Autodesk Inventor part; units mm, degrees
ref_plane "Płaszczyzna konstrukcyjna1" through (-3.5034, 3, 0) normal (0, 0, 1) x (1, 0, 0)
ref_plane "YZ Plane" through (0, 0, 0) normal (1, 0, 0) x (0, 1, 0)
ref_plane "XZ Plane" through (0, 0, 0) normal (0, 1, 0) x (-1, 0, 0)
sketch "Szkic1" plane through (0, 0, 0) normal (0, 1, 0) x (-1, 0, 0)
  line L0 (42.918, 0) -> (-17.7038, -35)
  line L1 (-17.7038, -35) -> (-17.7038, 35)
  line L2 (-17.7038, 35) -> (42.918, 0)
  point P0 (0, 0)
  dimension "d0" = 70
  dimension "d1" = 35
  dimension "d2" = 60
  dimension "d3" = 60
extrude "Wyciągnięcie proste1" add sketch "Szkic1" along normal blind 3
fillet "Zaokrąglenie1" radius 7 3 edges at (17.7038, 1.5, 35) (17.7038, 1.5, -35) (-42.918, 1.5, 0)
sketch "Szkic2" plane through (0, 3, 0) normal (0, 1, 0) x (1, 0, 0)
  circle A0 centre (10.92, -22.8756) radius 2.5
  arc A1 (7.2038, -28.9378) -> (17.7038, -22.8756) centre (10.7038, -22.8756) ccw
  circle A2 centre (-28.918, 0) radius 2.5
  circle A3 centre (10.7038, 23.0617) radius 2.5
  arc A4 (-32.418, 6.0622) -> (-32.418, -6.0622) centre (-28.918, 0) ccw
  arc A5 (17.7038, 22.8756) -> (7.2038, 28.9378) centre (10.7038, 22.8756) ccw
  point P0 (0, 0)
  dimension "d7" = 0
  dimension "d8" = 5
  dimension "d9" = 5
  dimension "d10" = 5
  dimension "d11" = 0
  dimension "d12" = 0
extrude "Wyciągnięcie proste2" cut sketch "Szkic2" against normal blind 3
sketch "Szkic3" plane through (0, 3, 0) normal (0, 1, 0) x (1, 0, 0)
  line L0 (7.2038, 28.9378) -> (-32.418, 6.0622)
  line L1 (-32.418, -6.0622) -> (7.2038, -28.9378)
  line L2 (7.2038, -28.9378) -> (-32.418, -6.0622)
  circle A0 centre (-2.5034, 0) radius 1
  point P0 (0, 0)
  point P1 (-12.6071, -17.5)
  point P2 (-12.6071, 17.5)
  dimension "d18" = 2
extrude "Wyciągnięcie proste3" cut sketch "Szkic3" against normal blind 3
sketch "Szkic4" plane through (-32.418, 0, 6.0622) normal (-0.5, 0, 0.866) x (0.866, 0, 0.5)
  point P0 (25.0437, 0)
sketch "Szkic5" plane through (0, 3, 0) normal (0, 1, 0) x (1, 0, 0)
  circle A0 centre (-2.5034, 0) radius 1
  line L0 (-3.5034, 0) -> (-3.5034, -1.2647)
  point P0 (0, 0)
  dimension "d19" = 1
ref_plane "Płaszczyzna konstrukcyjna1" through (-3.5034, 3, 0) normal (0, 0, 1) x (1, 0, 0)
sketch "Szkic6" plane through (0, 3, 0) normal (0, 1, 0) x (1, 0, 0)
  point P0 (0, 0)
sketch "Szkic7" plane through (-3.5034, 3, 0) normal (0, 0, 1) x (1, 0, 0)
  line L0 (0, 0) -> (2, 0)
  line L1 (1, 0) -> (-1.5981, 0)
  line L2 (1, -1.5) -> (-1.5981, 0)
  line L3 (1, -1.5) -> (1, 0)
  line L4 (1, 0.6) -> (1, -3.6)
  point P0 (3.5034, -3)
  dimension "d20" = 1.5
  dimension "d21" = 60
revolve "Obrót1" cut sketch "Szkic7" angle 360 about axis through (-2.5034, 3, 0) along (0, -1, 0)
sketch "Szkic8" plane through (0, 3, 0) normal (0, 1, 0) x (1, 0, 0)
  point P0 (0, 0)
properties part number "HandlePrimaryMirror" material "Aluminium 6061"
The listing builds one solid part. Answer for the finished solid, in the listing's coordinates (mm). Coordinates: 2 decimals unless noted, no trailing zeros. Order: outer loops, then holes, each group sorted by start corner. A loop starts at its lowest first (then second) coordinate and runs counter-clockwise, first axis right, second up. Notation, with made-up numbers: M 73.5,52.5 L 107.5,52.5 A14 ccw 107.5,59.5 Z; hole C -36,59.5 d5. An arc over 180 degrees is marked long. Answer as a JSON object with one key per item and string values. Group by question number.
1. Section B-B on y = 0.55 is taken. Write down the section's boundary in (x, z).
2. Section D-D on x = -14 is taken. Write down the section's boundary in (y, z), then the cut area to 3 significant figures.
3. Straight lines are drawn through the part: line 1 (X direction, y = 1.65, z = 0); line 2 (Z direction, x = 10.92, y = 2.35); line 3 (X direction, y = 1.55, z = -24.5). For each, find the intervals that lie inside material, in ascending order.
4. Determine the mould class of faces 1 (the flat face through (3, 3, 0)), 2 (the cylindrical face through (14.292, 1.521, -28.886)), 3 (the cylindrical face through (10.38, 1.52, -25.54)), 4 (the flat face through (-12.884, 1.479, -17.34)) for opening direction X: released by +X, released by -X, zero draft, split by the parting line, or undercut.
5. Flat-ended cylindrical pins translate along their axes: P1, Ø1.5, axis at x = 9, y = 1, coming from the -Z side; P2, Ø1.5, axis at y = 1.5, z = -8.5, coming from the -X side. Find the tip coordinate at first contact, or state that the pin passes through.
6. Section A-A on z = 0 is taken. Write down the section's boundary in (x, y).
7. Section C-C on x = 10.92 is taken. Write down the section's boundary in (y, z).
Values follow:
{
 "1": {"outline": "M -32.42,-6.06 L 7.2,-28.94 A7 ccw 17.7,-22.88 L 17.7,22.88 A7 ccw 7.2,28.94 L -32.42,6.06 A7 ccw Z; hole C -28.92,0 d5; hole C -2.5,0 d2; hole C 10.7,-23.06 d5; hole C 10.92,22.88 d5"},
 "2": {"outline": "M 0,-16.7 L 3,-16.7 L 3,16.7 L 0,16.7 Z", "area": "100 mm2"},
 "3": {"line 1": "-35.92 to -31.42, -26.42 to -3.5, -1.5 to 17.7", "line 2": "-29.87 to -25.55, -20.57 to 20.38, 25.38 to 29.87", "line 3": "-0.48 to 8.66, 12.75 to 17.51"},
 "4": {"face 1": "zero draft", "face 2": "split by the parting line", "face 3": "undercut", "face 4": "released by -X"},
 "5": {"P1": "z = -29.81", "P2": "x = -29.49"},
 "6": {"outline": "M -35.92,0 L -31.42,0 L -31.42,3 L -35.92,3 Z; M -26.42,0 L -3.5,0 L -3.5,2.08 L -5.1,3 L -26.42,3 Z; M -1.5,0 L 17.7,0 L 17.7,3 L 0.09,3 L -1.5,2.08 Z"},
 "7": {"outline": "M 0,-29.87 L 3,-29.87 L 3,-25.55 L 0,-25.55 Z; M 0,-20.57 L 3,-20.57 L 3,20.38 L 0,20.38 Z; M 0,25.38 L 3,25.38 L 3,29.87 L 0,29.87 Z"}
}
